Check sheet for the modelled part. Datum: model origin and axes. Units: mm. A direction names the side the tool comes from. Give positions to 0.01 mm unless a question says otherwise; leave off trailing zeros. Write each loop counter-clockwise with the first axis right and the second up, starting at its lowest first coordinate (ties: lowest second). Pieces come first, ordered by that corner, then holes. Notation, with made-up numbers: (17.25, -32) -> (50.25, -32) arc R21 ccw to (50.25, 2) -> close; hole circle Ø3 at (88, 1.5). An arc over 180 degrees is marked (long way). Answer as a JSON object with one key per item and string values.
from build123d import *

# Parameters (mm, degrees)
F0_R     = 44
F0_R_2   = 19
F1_DEPTH = 5
F2_R     = 33.75
F3_DEPTH = 2
F5_DEPTH = 25


with BuildPart() as f1:
    # F0 (on Front) → F1 (new body)
    with BuildSketch(Plane.XZ):
        Circle(F0_R)
        Circle(F0_R_2, mode=Mode.SUBTRACT)
    extrude(amount=F1_DEPTH)

    # F2 (on face) → F3 (cut)
    with BuildSketch(Plane.XZ.offset(5)):
        Circle(F2_R)
    extrude(amount=-F3_DEPTH, mode=Mode.SUBTRACT)

    # F4 (on Front) → F5 (cut)
    with BuildSketch(Plane.XZ):
        Polygon((-49.323015, 0), (0, 0), (50.371692, 0), (50.371692, 35.833221), (0, 51.775392), (-49.323015, 41.89574), align=None)
    extrude(amount=F5_DEPTH, mode=Mode.SUBTRACT)


solid = f1.part
1. Go/stop test with flat-tipped pins: P1, Ø3, axis at x = 12.5, y = -3.5, coming from the +Z side; P2, Ø1.5, axis at y = -2.5, z = -32.5, coming from the -X side; P3, Ø12, axis at x = -13.5, z = -17, coming from the -Y side. Record where each tip stops, or that it passes through.
Determined:
{"P1": "z = -12.94", "P2": "x = -30.46", "P3": "y = -3"}
2. Sectioned sample at D-D, the plane x = -11.5. Enter the section's corners in (y, z).
Determined:
{"outline": "(-5, -42.47) -> (0, -42.47) -> (0, -15.12) -> (-3, -15.12) -> (-3, -31.73) -> (-5, -31.73) -> close"}
3. Sectioned sample at B-B, the plane x = 0. Enter the section's corners in (y, z), plus the area to 3 significant figures.
Determined:
{"outline": "(-5, -44) -> (0, -44) -> (0, -19) -> (-3, -19) -> (-3, -33.75) -> (-5, -33.75) -> close", "area": "95.5 mm^2"}
4. Access from +Z, -Z, +X, -X, +Y, -Y to the whole of each face (thin tool, end or side, straight path). Record for faces 4 (the face through (0, -1, -19)), 5 (the face through (-0.74, -4.01, -33.74)).
Determined:
{"face 4": "+Z, +Y, -Y", "face 5": "+Z, -Y"}
5. Scan lines: L1, parallel to Y at x = 7, z = -31.5; L2, parallel to X at y = -3.35, z = -14; L3, parallel to X at y = -1.5, z = -8. Record each from-to range of solid material in increasing order. Write a range as [from, to].
Determined:
{"L1": "[-3, 0]", "L2": "[-41.71, -30.71], [30.71, 41.71]", "L3": "[-43.27, -17.23], [17.23, 43.27]"}
6. Sectioned sample at A-A, the plane z = -13. Enter the section's corners in (x, y).
Determined:
{"outline": "(-42.04, -5) -> (-31.15, -5) -> (-31.15, -3) -> (-13.86, -3) -> (-13.86, 0) -> (-42.04, 0) -> close; (13.86, -3) -> (31.15, -3) -> (31.15, -5) -> (42.04, -5) -> (42.04, 0) -> (13.86, 0) -> close"}
7. Sectioned sample at C-C, the plane y = -3.9. Enter the section's corners in (x, z), plus the area to 3 significant figures.
Determined:
{"outline": "(-44, 0) arc R44 ccw to (44, 0) -> (33.75, 0) arc R33.75 cw to (-33.75, 0) -> close", "area": "1,250 mm^2"}
8. Mould release check, pull along X, two halves, no side actions. Record for faces 1 (the face through (0, -3, -20)), 2 (the face through (-0.97, -2.46, -43.99)), 3 (the face through (-6.7, -5, -33.3)): released by +X, released by -X, zero draft, split by the parting line, or undercut.
Determined:
{"face 1": "undercut", "face 2": "split by the parting line", "face 3": "zero draft"}
